Can you work these out from the model? Positions are in its coordinate system, mm. Face numbers are marked on the shaded views. A direction names the side the tool comes from. Give positions to 0.01 mm unless a question says otherwise; leave off trailing zeros. Order: outer loops, then holes, each group sorted by start corner. A loop starts at its lowest first (then second) coordinate and runs counter-clockwise, first axis right, second up.
Item 1: I'm going to push flat-ended pins straight in: pin 1 Ø12 at (x, y) = (-48, 74) entering from -Z; pin 2 Ø5 at (x, y) = (-22.5, -56) entering from -Z; pin 3 Ø2 at (x, z) = (-10.5, -7.5) entering from -Y. Where does each tip first touch, or does it pass through?
Item 2: I want a section at A-A, the plane z = 25. Write out the boundary of the cut face in (x, y), then the cut area to 3 significant figures.
Item 3: I want a section at B-B, the plane z = -10. Write out the boundary of the cut face in (x, y).
Item 4: Which directions (+Z, -Z, +X, -X, +Y, -Y) give clear straight access to the entire face, cutting with the end or side of a thin tool? Please do the marked faces 1 and 2.
Item 5: If I drill on line 1 along Y through (x, z) = (0, 2.85); line 2 along Z through (x, y) = (39, -70); line 3 along Z through (x, y) = (-19.5, 45.5), over which ranges is the centre line in solid material (lowest first)?
```python
from build123d import *

# Parameters (mm, degrees)
SKETCH002_R = 1.5
HOLE_DEPTH  = 25
HOLE_TIPS_R = 1.5


with BuildPart() as part:
    # Sketch → Revolution (revolve)
    with BuildSketch(Plane.XZ):
        with BuildLine():
            Line((0, 0), (50, 0))
            ThreePointArc((50, 0), (109.895652, 2.5), (50, 5))
            Line((50, 5), (0, 5))
            Line((0, 5), (0, 0))
        make_face()
    revolve(axis=Axis((0, 0, 0), (0, 0, 1)))

    # Sketch002 (on Face3 of Revolution) → Hole (cut)
    with BuildSketch(Plane(origin=(0, 0, 5), x_dir=(-1, 0, 0), z_dir=(0, 0, 1))):
        Circle(SKETCH002_R)
    extrude(amount=-HOLE_DEPTH, mode=Mode.SUBTRACT)

    # Hole tips → Hole tip 1 section 0
    with BuildSketch(Plane(origin=(0, 0, -20), x_dir=(-1, 0, 0), z_dir=(0, 0, 1)), mode=Mode.PRIVATE) as hole_tip_1_s0:
        Circle(HOLE_TIPS_R)
    loft([hole_tip_1_s0.sketch, Vertex(0, 0, -20.901291)], mode=Mode.SUBTRACT)


solid = part.part
```
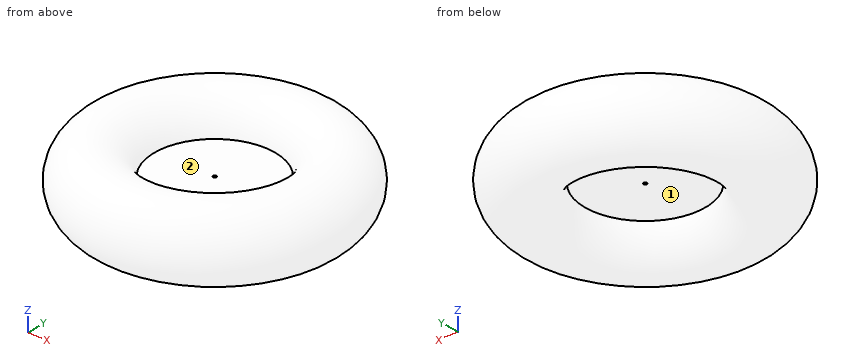
Results list:
1. pin 1: stops at z = -27.41
1. pin 2: stops at z = -22.19
1. pin 3: stops at y = -108.02
2. outline: circle Ø199.48 at (0, 0); hole circle Ø120.11 at (0, 0)
2. area: 19,900 mm2
3. outline: circle Ø214.33 at (0, 0); hole circle Ø105.25 at (0, 0)
4. face 1: -Z
4. face 2: +Z
5. line 1: y = -109.89 to -1.5, 1.5 to 109.89
5. line 2: z = -27.5 to 32.5
5. line 3: z = 0 to 5
